```python
from build123d import *

# Parameters (mm, degrees)
SKETCH1_R           = 89
BOSS_EXTRUDE1_DEPTH = 8
SKETCH2_R           = 80
BOSS_EXTRUDE2_DEPTH = 40
CHAMFER2_SIZE       = 30
SKETCH5_R           = 45.325276546
BOSS_EXTRUDE3_DEPTH = 26
SKETCH6_R           = 2.574541915
CUT_EXTRUDE1_DEPTH  = 26


with BuildPart() as part:
    # Sketch1 → Boss-Extrude1 (new body)
    with BuildSketch(Plane.XY):
        Circle(SKETCH1_R)
    extrude(amount=BOSS_EXTRUDE1_DEPTH)

    # Sketch2 → Boss-Extrude2 (add)
    with BuildSketch(Plane.XY.offset(8)):
        Circle(SKETCH2_R)
    extrude(amount=BOSS_EXTRUDE2_DEPTH)

    # Chamfer2
    chamfer2_edges = [part.edges().sort_by_distance(p)[0] for p in [
        (-80, 0, 48),
    ]]
    chamfer(chamfer2_edges, length=CHAMFER2_SIZE)

    # Sketch5 → Boss-Extrude3 (add)
    with BuildSketch(Plane.XY.offset(48)):
        Circle(SKETCH5_R)
    extrude(amount=BOSS_EXTRUDE3_DEPTH)

    # Sketch6 → Cut-Extrude1 (cut)
    with BuildSketch(Plane.XY.offset(8)):
        with Locations((0, 84.547956484)):
            Circle(SKETCH6_R)
        with Locations((84.547956484, 0)):
            Circle(SKETCH6_R)
        with Locations((0, -84.547956484)):
            Circle(SKETCH6_R)
        with Locations((-84.547956484, 0)):
            Circle(SKETCH6_R)
    extrude(amount=-CUT_EXTRUDE1_DEPTH, mode=Mode.SUBTRACT)


solid = part.part
```
For this review, take the finished solid that the model builds, in its own axes (mm). A direction names the side the tool comes from. Round coordinates to 2 decimals unless told otherwise and drop trailing zeros. Order: outer loops, then holes, each group sorted by start corner. A loop starts at its lowest first (then second) coordinate and runs counter-clockwise, first axis right, second up.
Q1. We need section D-D, the plane z = 23.5. Give the boundary of the cut face in (x, y), plus the area to 3 significant figures.
Findings below:
outline: circle Ø149 at (0, 0)
area: 17,400 mm2
Q2. Insertion check: P1, Ø6, axis at y = -28, z = 39, coming from the -X side; P2, Ø4, axis at x = 0, y = -84.55, coming from the -Z side; P3, Ø6.5, axis at x = -84.55, y = 0, coming from the +Z side; P4, Ø5, axis at x = 19, z = 39, coming from the -Y side. Each pin has a flat end and moves straight along its axis. Give the tip position at first contact, or say it passes through.
Findings below:
P1: stops at x = -55.63
P2: passes through
P3: stops at z = 8
P4: stops at y = -58.61
Q3. Wall thickness on line 1 (Z direction, x = -45.5, y = -67); line 2 (X direction, y = 12.5, z = 49.5); line 3 (Y direction, x = -4.5, z = 58): over which ranges is each line inside the solid? List them lowest first.
Findings below:
line 1: z = 0 to 8
line 2: x = -43.57 to 43.57
line 3: y = -45.1 to 45.1
Q4. We need section C-C, the plane z = 50.5. Give the boundary of the cut face in (x, y).
Findings below:
outline: circle Ø90.65 at (0, 0)
Q5. Mouldability with a two-part tool opening along X and no side actions: class faces 1 (the flat face through (-1, 1, 74)), 2 (the cylindrical face through (-65.597, 60.15, 3.944)), 3 (the cylindrical face through (-0.335, -81.995, 4.056)), 4 (the cylindrical face through (-82.17, -0.99, 4.06)) as pulls with the +X half, pulls with the -X half, needs draft (parallel to the pull), parting line crosses it, or undercut.
Findings below:
face 1: needs draft
face 2: parting line crosses it
face 3: undercut
face 4: undercut
Q6. Machinability: for faces 5 (the cylindrical face through (81.976, 0.113, 4.056)), 6 (the cylindrical face through (-17.34, -78.1, 12.93)), which of the approach directions +Z, -Z, +X, -X, +Y, -Y give a long, thin tool a straight path to every point of the face, cutting with its end or side? Answer none if there is none.
Findings below:
face 5: +Z, -Z
face 6: +Z
Q7. We need section A-A, the plane y = 0. Give the boundary of the cut face in (x, z), plus the area to 3 significant figures.
Findings below:
outline: (-89, 0) - (-87.12, 0) - (-87.12, 8) - (-89, 8) - close; (-81.97, 0) - (81.97, 0) - (81.97, 8) - (80, 8) - (80, 18) - (50, 48) - (45.33, 48) - (45.33, 74) - (-45.33, 74) - (-45.33, 48) - (-50, 48) - (-80, 18) - (-80, 8) - (-81.97, 8) - close; (87.12, 0) - (89, 0) - (89, 8) - (87.12, 8) - close
area: 9,200 mm2
